```python
from build123d import *

# Parameters (mm, degrees)
SKETCH1_W           = 35
SKETCH1_H           = 120
BOSS_EXTRUDE1_DEPTH = 7.5
SKETCH2_W           = 32.5
SKETCH2_H           = 2.5
BOSS_EXTRUDE2_DEPTH = 20
SKETCH3_R           = 1.4
CUT_EXTRUDE1_DEPTH  = 12
SKETCH4_R           = 2.95
BOSS_EXTRUDE3_DEPTH = 4


with BuildPart() as part:
    # Sketch1 → Boss-Extrude1 (new body)
    with BuildSketch(Plane(origin=(0, 0, 0), x_dir=(1, 0, 0), z_dir=(0, 1, 0))):
        with Locations((17.5, 0)):
            Rectangle(SKETCH1_W, SKETCH1_H)
    extrude(amount=BOSS_EXTRUDE1_DEPTH)

    # Sketch2 → Boss-Extrude2 (add)
    with BuildSketch(Plane(origin=(0, 7.5, 0), x_dir=(1, 0, 0), z_dir=(0, 1, 0))):
        Polygon((35, 2.55), (35, 60), (32.5, 60), (32.5, 5.05), (32.5, 2.55), align=None)
        with Locations((16.25, 3.8)):
            Rectangle(SKETCH2_W, SKETCH2_H)
        with Locations((16.25, -3.8)):
            Rectangle(SKETCH2_W, SKETCH2_H)
        Polygon((35, -60), (35, -2.55), (32.5, -2.55), (32.5, -5.05), (32.5, -60), align=None)
    extrude(amount=BOSS_EXTRUDE2_DEPTH)

    # Sketch3 → Cut-Extrude1 (cut)
    with BuildSketch(Plane.XY.offset(5.05)):
        with Locations((5, 25)):
            Circle(SKETCH3_R)
        with Locations((5, 15)):
            Circle(SKETCH3_R)
        with Locations((20, 25)):
            Circle(SKETCH3_R)
        with Locations((20, 15)):
            Circle(SKETCH3_R)
    extrude(amount=-CUT_EXTRUDE1_DEPTH, mode=Mode.SUBTRACT)

    # Sketch4 → Boss-Extrude3 (add)
    with BuildSketch(Plane(origin=(35, 0, 0), x_dir=(0, 0, -1), z_dir=(1, 0, 0))):
        with Locations(Location((-48, 17.5, 0), (0, 0, 180))):
            Circle(SKETCH4_R)
        with Locations(Location((48, 17.5, 0), (0, 0, 180))):
            Circle(SKETCH4_R)
    extrude(amount=BOSS_EXTRUDE3_DEPTH)


solid = part.part
```
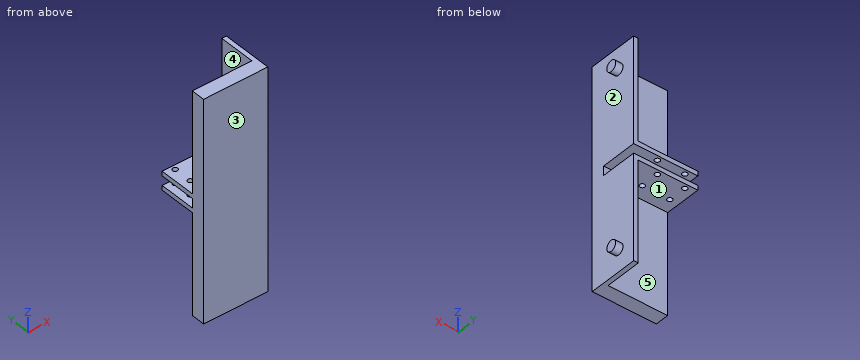
Input: part model. Units: mm. Frame: model coordinates. Face numbers are marked on the shaded views. A direction names the side the tool comes from. Coordinates: 2 decimals unless noted, no trailing zeros. Loops run counter-clockwise (first coordinate to the right, second up) from the corner with the lowest first, then second, coordinate; pieces in that order, holes last. Notation, with made-up numbers: (79.25, -29) - (85.25, -29) arc R27 cw to (85.25, 3) - close; hole circle Ø8 at (51.5, -0.75). An arc over 180 degrees is marked (long way). Answer in a Markdown table with one row per item.
(1) Mould query, pull axis Z, two halves, no side actions, for the marked faces 1, 2 and 3. Classes: pulls with the +Z half, pulls with the -Z half, needs draft (parallel to the pull), parting line crosses it, or undercut.
Model answer:
| item | result |
|---|---|
| face 1 | pulls with the -Z half |
| face 2 | undercut |
| face 3 | needs draft |
(2) Cut plane C-C on z = 48. Output: boundary loops of the cut face in (x, y).
Model answer:
| item | result |
|---|---|
| outline | (0, 0) - (35, 0) - (35, 14.55) - (39, 14.55) - (39, 20.45) - (35, 20.45) - (35, 27.5) - (32.5, 27.5) - (32.5, 7.5) - (0, 7.5) - close |
(3) Pin query (flat end, axial travel): P1, Ø1.7, axis at x = 5, y = 25, coming from the +Z side; P2, Ø8, axis at x = 8, z = 39, coming from the -Y side; P3, Ø3.5, axis at x = 20, y = 15, coming from the +Z side; P4, Ø10, axis at x = 7.5, y = 16, coming from the -Z side. Return the tip coordinate at first contact, or that it passes through.
Model answer:
| item | result |
|---|---|
| P1 | passes through |
| P2 | stops at y = 0 |
| P3 | stops at z = 5.05 |
| P4 | stops at z = -5.05 |
(4) Cut plane D-D on z = 19. Output: boundary loops of the cut face in (x, y).
Model answer:
| item | result |
|---|---|
| outline | (0, 0) - (35, 0) - (35, 27.5) - (32.5, 27.5) - (32.5, 7.5) - (0, 7.5) - close |
(5) Cut plane B-B on x = 5. Output: boundary loops of the cut face in (y, z).
Model answer:
| item | result |
|---|---|
| outline | (0, -60) - (7.5, -60) - (7.5, -5.05) - (13.6, -5.05) - (13.6, -2.55) - (7.5, -2.55) - (7.5, 2.55) - (13.6, 2.55) - (13.6, 5.05) - (7.5, 5.05) - (7.5, 60) - (0, 60) - close; (16.4, -5.05) - (23.6, -5.05) - (23.6, -2.55) - (16.4, -2.55) - close; (16.4, 2.55) - (23.6, 2.55) - (23.6, 5.05) - (16.4, 5.05) - close; (26.4, -5.05) - (27.5, -5.05) - (27.5, -2.55) - (26.4, -2.55) - close; (26.4, 2.55) - (27.5, 2.55) - (27.5, 5.05) - (26.4, 5.05) - close |
(6) Material intervals for L1, parallel to Y at x = 20, z = 4; L2, parallel to Z at x = 26, y = 25.5; L3, parallel to Y at x = 5, z = 22, sorted ascending. Write a range as from..to.
Model answer:
| item | result |
|---|---|
| L1 | y = 0..13.6, 16.4..23.6, 26.4..27.5 |
| L2 | z = -5.05..-2.55, 2.55..5.05 |
| L3 | y = 0..7.5 |
(7) Cut plane A-A on y = 25. Output: boundary loops of the cut face in (x, z).
Model answer:
| item | result |
|---|---|
| outline | (0, -5.05) - (3.6, -5.05) - (3.6, -2.55) - (0, -2.55) - close; (0, 2.55) - (3.6, 2.55) - (3.6, 5.05) - (0, 5.05) - close; (6.4, -5.05) - (18.6, -5.05) - (18.6, -2.55) - (6.4, -2.55) - close; (6.4, 2.55) - (18.6, 2.55) - (18.6, 5.05) - (6.4, 5.05) - close; (21.4, -5.05) - (32.5, -5.05) - (32.5, -60) - (35, -60) - (35, -2.55) - (21.4, -2.55) - close; (21.4, 2.55) - (35, 2.55) - (35, 60) - (32.5, 60) - (32.5, 5.05) - (21.4, 5.05) - close |
(8) Set-up query: the marked faces 4 and 5. Return all of +Z, -Z, +X, -X, +Y, -Y with unobstructed straight access to the full face (end or side cutting, diameter ignored); none if empty.
Model answer:
| item | result |
|---|---|
| face 4 | +Z, -X, +Y |
| face 5 | -Z, -X, +Y |
